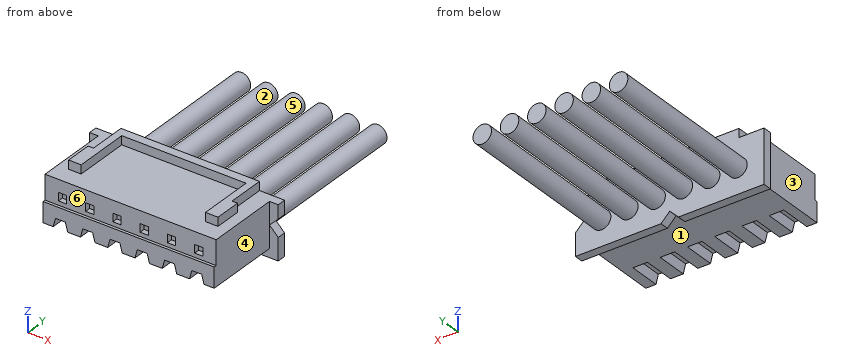
```python
from build123d import *

# Parameters (mm, degrees)
ESQUISSE1_W                = 15.7
ESQUISSE1_H                = 4.1
BOSS_EXTRU_1_DEPTH         = 7.75
ESQUISSE2_W                = 15.7
ESQUISSE2_H                = 2.25
ENL_V_MAT_EXTRU_1_DEPTH    = 0.25
ESQUISSE3_W                = 17.3
ESQUISSE3_H                = 4.9
BOSS_EXTRU_2_DEPTH         = 0.8
ENL_V_MAT_EXTRU_4_DEPTH    = 12.95857433
BOSS_EXTRU_3_DEPTH         = 0.8
ENL_V_MAT_EXTRU_2_DEPTH    = 2.9
ESQUISSE6_W                = 0.75
ESQUISSE6_H                = 0.75
ENL_V_MAT_EXTRU_3_DEPTH    = 0.5
ESQUISSE7_R                = 0.85
BOSS_EXTRU_4_DEPTH         = 15
R_P_TITION_LIN_AIRE2_COUNT = 6
R_P_TITION_LIN_AIRE2_PITCH = 2.5


with BuildPart() as part:
    # Esquisse1 → Boss.-Extru.1 (new body)
    with BuildSketch(Plane(origin=(0, 0, 0), x_dir=(1, 0, 0), z_dir=(0, 1, 0))):
        Rectangle(ESQUISSE1_W, ESQUISSE1_H)
    extrude(amount=BOSS_EXTRU_1_DEPTH)

    # Esquisse2 → Enlèv. mat.-Extru.1 (cut)
    with BuildSketch(Plane(origin=(0, 0, 0), x_dir=(1, 0, 0), z_dir=(0, 1, 0))):
        with Locations((0, -0.925)):
            Rectangle(ESQUISSE2_W, ESQUISSE2_H)
    extrude(amount=ENL_V_MAT_EXTRU_1_DEPTH, mode=Mode.SUBTRACT)

    # Esquisse3 → Boss.-Extru.2 (add)
    with BuildSketch(Plane(origin=(0, 7.75, 0), x_dir=(1, 0, 0), z_dir=(0, 1, 0))):
        with Locations((0, 0.4)):
            Rectangle(ESQUISSE3_W, ESQUISSE3_H)
    extrude(amount=-BOSS_EXTRU_2_DEPTH)

    # Esquisse8 → Enlèv. mat.-Extru.4 (cut, through all)
    with BuildSketch(Plane(origin=(0, 7.75, 0), x_dir=(1, 0, 0), z_dir=(0, 1, 0))):
        Polygon((-0.8, 2.85), (0, 2.05), (0.8, 2.85), align=None)
        Polygon((8.65, 0.8), (7.85, 0), (8.65, -0.8), align=None)
    extrude(amount=-ENL_V_MAT_EXTRU_4_DEPTH, mode=Mode.SUBTRACT)

    # Esquisse4 → Boss.-Extru.3 (add)
    with BuildSketch(Plane.XY.offset(2.05)):
        Polygon((5.7, 6.95), (-5.7, 6.95), (-5.7, 1.85), (-6.85, 1.85), (-6.85, 4.3), (-6.35, 4.3), (-6.35, 7.75), (6.35, 7.75), (6.35, 4.3), (6.85, 4.3), (6.85, 1.85), (5.7, 1.85), align=None)
    extrude(amount=BOSS_EXTRU_3_DEPTH)

    # Esquisse5 → Enlèv. mat.-Extru.2 (cut)
    with BuildSketch(Plane(origin=(0, 0, 0), x_dir=(1, 0, 0), z_dir=(0, 1, 0))):
        Polygon((-6.915, 2.05), (-6.7, 1.25), (-5.8, 1.25), (-5.585, 2.05), align=None)
    enl_v_mat_extru_2 = extrude(amount=ENL_V_MAT_EXTRU_2_DEPTH, mode=Mode.SUBTRACT)

    # Esquisse6 → Enlèv. mat.-Extru.3 (cut)
    with BuildSketch(Plane.XZ.offset(-0.25)):
        with Locations((-6.25, 0.545)):
            Rectangle(ESQUISSE6_W, ESQUISSE6_H)
    enl_v_mat_extru_3 = extrude(amount=-ENL_V_MAT_EXTRU_3_DEPTH, mode=Mode.SUBTRACT)

    # Esquisse7 → Boss.-Extru.4 (add)
    with BuildSketch(Plane(origin=(0, 7.75, 0), x_dir=(1, 0, 0), z_dir=(0, 1, 0))):
        with Locations(Location((-6.25, 0.554746523, 0), (0, 0, 270))):
            Circle(ESQUISSE7_R)
    boss_extru_4 = extrude(amount=BOSS_EXTRU_4_DEPTH)

    # Répétition linéaire2: Enlèv. mat.-Extru.2, Enlèv. mat.-Extru.3, Boss.-Extru.4 ×6
    with Locations(*[(i * R_P_TITION_LIN_AIRE2_PITCH, 0, 0) for i in range(1, R_P_TITION_LIN_AIRE2_COUNT)]):
        add(enl_v_mat_extru_2, mode=Mode.SUBTRACT)
        add(enl_v_mat_extru_3, mode=Mode.SUBTRACT)
        add(boss_extru_4)


solid = part.part
```
Model file for the job. Use its own axes, mm. Face numbers are marked on the shaded views. A direction names the side the tool comes from. Give positions to 0.01 mm unless a question says otherwise; leave off trailing zeros. Loops run counter-clockwise (first coordinate to the right, second up) from the corner with the lowest first, then second, coordinate; pieces in that order, holes last. Notation, with made-up numbers: (72, 28.25) -> (96, 28.25) arc R35 ccw to (96, 64.25) -> close; hole circle Ø3 at (7.25, 85). An arc over 180 degrees is marked (long way). Write each question's results on one line, items separated by ' | '.
(1) Pull direction X, two halves, no side cores. Call the marked faces 4, 5 and 6: released by +X, released by -X, zero draft, split by the parting line, or undercut.
Geometry results:
face 4: released by +X | face 5: undercut | face 6: zero draft
(2) Tool access for the marked faces 1, 2 and 3: list every direction of +Z, -Z, +X, -X, +Y, -Y with a clear straight run to the whole face (end or side of a thin tool).
Geometry results:
face 1: -Z, +X, -X, -Y | face 2: +Y | face 3: +Z, -Z, -X, -Y
(3) Cut at C-C on x = -5. List the corners of the cut face in (y, z).
Geometry results:
outline: (0, -2.05) -> (6.95, -2.05) -> (6.95, -2.85) -> (7.75, -2.85) -> (7.75, 2.85) -> (6.95, 2.85) -> (6.95, 2.05) -> (0.25, 2.05) -> (0.25, -0.2) -> (0, -0.2) -> close
(4) Cut at B-B on y = 17.5. List the corners of the cut face in (x, z), and give its area (3 significant figures).
Geometry results:
outline: circle Ø1.7 at (-6.25, -0.55); circle Ø1.7 at (-3.75, -0.55); circle Ø1.7 at (-1.25, -0.55); circle Ø1.7 at (1.25, -0.55); circle Ø1.7 at (3.75, -0.55); circle Ø1.7 at (6.25, -0.55) | area: 13.6 mm²
(5) Cut at D-D on x = 3.75. List the corners of the cut face in (y, z), and give its area (3 significant figures).
Geometry results:
outline: (0, -1.25) -> (2.9, -1.25) -> (2.9, -2.05) -> (6.95, -2.05) -> (6.95, -2.85) -> (7.75, -2.85) -> (7.75, -1.4) -> (22.75, -1.4) -> (22.75, 0.3) -> (7.75, 0.3) -> (7.75, 2.85) -> (6.95, 2.85) -> (6.95, 2.05) -> (0.25, 2.05) -> (0.25, 0.92) -> (0.75, 0.92) -> (0.75, 0.17) -> (0.25, 0.17) -> (0.25, -0.2) -> (0, -0.2) -> close | area: 55.3 mm²
(6) Probe line 1 along X through (y, z) = (18.5, 0.1); line 2 along X through (y, z) = (8.5, -1); line 3 along Y through (x, z) = (-7.5, 0.4). List the from-to ranges inside material, lowest first.
Geometry results:
line 1: x = -6.79 to -5.71, -4.29 to -3.21, -1.79 to -0.71, 0.71 to 1.79, 3.21 to 4.29, 5.71 to 6.79 | line 2: x = -6.97 to -5.53, -4.47 to -3.03, -1.97 to -0.53, 0.53 to 1.97, 3.03 to 4.47, 5.53 to 6.97 | line 3: y = 0.25 to 7.75
(7) Flat gauge pins, fed straight in: pin 1 Ø0.6 at (x, z) = (6.5, 0.5) entering from -Y; pin 2 Ø4 at (x, y) = (-2.5, 4.5) entering from -Z; pin 3 Ø0.6 at (y, z) = (6.5, 2.5) entering from -X. Where does each tip first touch, or does it go through?
Geometry results:
pin 1: stops at y = 0.25 | pin 2: stops at z = -2.05 | pin 3: stops at x = -6.35
(8) Cut at A-A on z = -2.35. List the corners of the cut face in (x, y).
Geometry results:
outline: (-8.65, 6.95) -> (-0.3, 6.95) -> (-0.3, 7.75) -> (-8.65, 7.75) -> close; (0.3, 6.95) -> (8.65, 6.95) -> (8.65, 7.75) -> (0.3, 7.75) -> close
